Geometry check sheet. Reference: the model listing, model coordinates, mm. Coordinates: 2 decimals unless noted, no trailing zeros. Order: outer loops, then holes, each group sorted by start corner. A loop starts at its lowest first (then second) coordinate and runs counter-clockwise, first axis right, second up. Notation, with made-up numbers: (12, -18) - (22, -18) arc R23 cw to (22, 7) - close; hole circle Ø4 at (4.25, 21). An arc over 180 degrees is marked (long way). Use CSV: the item, a comma, the result in double quotes. Start each with the question number.
1) Thickness scan on probe 1 along Z at (x, y) = (0, 34); probe 2 along Y at (x, z) = (9.5, 9); probe 3 along Z at (x, y) = (11, 26.5). Record the ranges inside material, lowest first. Write a range as [from, to].
2) Sectioned sample at C-C, the plane y = 47.5. Record the cut outline in (x, z), and give its area (3 significant figures).
3) Depth check by flat-ended pin: P1, Ø4, axis at y = 28.5, z = 16, coming from the -X side; P2, Ø5, axis at y = 26, z = -11, coming from the -X side; P3, Ø3, axis at x = -12.5, y = 19, coming from the -Z side. Enter the tip coordinate at first touch or a pass-through.
4) Sectioned sample at B-B, the plane x = 0. Record the cut outline in (y, z).
5) Sectioned sample at A-A, the plane z = 0. Record the cut outline in (x, y), and give its area (3 significant figures).
6) Draft check along X on faces 1 (the flat face through (0, 0, 0)), 2 (the cylindrical face through (-10.382, 46.835, 19.961)), 3 (the flat face through (-17, 95, -15)). Enter one of: released by +X, released by -X, zero draft, split by the parting line, or undercut.
Autodesk Inventor part; units mm, degrees
ref_plane "YZ Plane" through (0, 0, 0) normal (1, 0, 0) x (0, 1, 0)
ref_plane "XZ Plane" through (0, 0, 0) normal (0, 1, 0) x (-1, 0, 0)
ref_plane "XY Plane" through (0, 0, 0) normal (0, 0, 1) x (1, 0, 0)
sketch "Sketch1" plane through (0, 0, 0) normal (0, 1, 0) x (-1, 0, 0)
  circle A0 centre (0, 0) radius 22.5
  circle A1 centre (0, 0) radius 23
  dimension "d0" = 45
  dimension "d1" = 46
extrude "Extrusion1" add sketch "Sketch1" along normal blind 95
sketch "Sketch2" plane through (0, 0, 0) normal (0, -1, 0) x (1, 0, 0)
  circle A0 centre (0, 0) radius 23
  circle A1 centre (0, -23) radius 0.5
  dimension "d8" = 1
sketch "Sketch3" plane through (0, 0, 0) normal (0, -1, 0) x (1, 0, 0)
  circle A0 centre (0, 0) radius 23
  dimension "d4" = 46
extrude "Extrusion2" add sketch "Sketch3" along normal blind 1
fillet "Fillet1" radius 1 1 edges at (-23, -1, 0)
properties part number "Dalek Light 2"
Evaluation:
1,probe 1,"[-23, -22.5], [22.5, 23]"
1,probe 2,"[-1, 0]"
1,probe 3,"[-20.2, -19.63], [19.63, 20.2]"
2,outline,"circle Ø46 at (0, 0); hole circle Ø45 at (0, 0)"
2,area,"71.5 mm²"
3,P1,"x = -18.25"
3,P2,"x = -21.37"
3,P3,"z = -20.2"
4,outline,"(-1, -22) arc R1 ccw to (0, -23) - (95, -23) - (95, -22.5) - (0, -22.5) - (0, 22.5) - (95, 22.5) - (95, 23) - (0, 23) arc R1 ccw to (-1, 22) - close"
5,outline,"(-23, 0) arc R1 ccw to (-22, -1) - (22, -1) arc R1 ccw to (23, 0) - (23, 95) - (22.5, 95) - (22.5, 0) - (-22.5, 0) - (-22.5, 95) - (-23, 95) - close"
5,area,"141 mm²"
6,face 1,"undercut"
6,face 2,"undercut"
6,face 3,"zero draft"
